from build123d import *

# Parameters (mm, degrees)
SALIENTE_EXTRUIR1_DEPTH = 50
CROQUIS3_R              = 1.75
CORTAR_EXTRUIR1_DEPTH   = 50
CORTAR_EXTRUIR2_DEPTH   = 50
CROQUIS5_W              = 13.75
CROQUIS5_H              = 15.668518787
SALIENTE_EXTRUIR2_DEPTH = 5
CROQUIS6_R              = 3.25
CORTAR_EXTRUIR3_DEPTH   = 51


with BuildPart() as part:
    # Croquis1 → Saliente-Extruir1 (new body)
    with BuildSketch(Plane.XY):
        Polygon((-11.139985082, 4.35106383), (12.860014918, 4.35106383), (8.360014918, 22.35106383), (-6.639985082, 22.35106383), align=None)
        Polygon((-6.068188312, 13.064935956), (-2.604086697, 7.064935956), (4.324116534, 7.064935956), (7.788218149, 13.064935956), (4.324116534, 19.064935956), (-2.604086697, 19.064935956), align=None, mode=Mode.SUBTRACT)
    extrude(amount=SALIENTE_EXTRUIR1_DEPTH)

    # Croquis3 → Cortar-Extruir1 (cut)
    with BuildSketch(Plane.XZ.offset(-4.35106383)):
        with Locations((-8.139985082, 3.5)):
            Circle(CROQUIS3_R)
        with Locations((9.860014918, 46.5)):
            Circle(CROQUIS3_R)
    extrude(amount=-CORTAR_EXTRUIR1_DEPTH, mode=Mode.SUBTRACT)

    # Croquis4 → Cortar-Extruir2 (cut)
    with BuildSketch(Plane(origin=(0, 7.35106383, 0), x_dir=(-1, 0, 0), z_dir=(0, -1, 0))):
        with BuildLine():
            Line((-18.110014918, -43.75), (-9.860014918, -43.75))
            ThreePointArc((-9.860014918, -43.75), (-7.91547127, -44.555456352), (-7.110014918, -46.5))
            Line((-7.110014918, -46.5), (-7.110014918, -54.75))
            Line((-7.110014918, -54.75), (-18.110014918, -54.75))
            Line((-18.110014918, -54.75), (-18.110014918, -43.75))
        make_face()
        with BuildLine():
            Line((16.389985082, -6.25), (8.139985082, -6.25))
            ThreePointArc((8.139985082, -6.25), (6.195441433, -5.444543648), (5.389985082, -3.5))
            Line((5.389985082, -3.5), (5.389985082, 4.75))
            Line((5.389985082, 4.75), (16.389985082, 4.75))
            Line((16.389985082, 4.75), (16.389985082, -6.25))
        make_face()
    extrude(amount=-CORTAR_EXTRUIR2_DEPTH, mode=Mode.SUBTRACT)

    # Croquis5 → Saliente-Extruir2 (add)
    with BuildSketch(Plane.XY.offset(50)):
        with Locations((0.235014918, 14.516804437)):
            Rectangle(CROQUIS5_W, CROQUIS5_H)
    extrude(amount=-SALIENTE_EXTRUIR2_DEPTH)

    # Croquis6 → Cortar-Extruir3 (cut, through all)
    with BuildSketch(Plane(origin=(0, 0, 0), x_dir=(-1, 0, 0), z_dir=(0, 0, -1))):
        with Locations((-0.860014918, 12.564935956)):
            Circle(CROQUIS6_R)
    extrude(amount=-CORTAR_EXTRUIR3_DEPTH, mode=Mode.SUBTRACT)


solid = part.part
Design review of the part built by this model. Coordinates are the model's own, in mm. A direction names the side the tool comes from. Coordinates: 2 decimals unless noted, no trailing zeros. Loops run counter-clockwise (first coordinate to the right, second up) from the corner with the lowest first, then second, coordinate; pieces in that order, holes last. Notation, with made-up numbers: (82, 64) -> (118, 64) arc R30 cw to (118, 101) -> close; hole circle Ø4 at (-9.5, 89). An arc over 180 degrees is marked (long way). Use a Markdown table: item, result. Add a question column.
Item 1: Wall thickness on L1, parallel to Y at x = -2.5, z = 34; L2, parallel to Z at x = -3, y = 12.75; L3, parallel to Z at x = -8.75, y = 12.5: over which ranges is each line inside the solid? List them lowest first. Write a range as from..to.
Item 2: We need section A-A, the plane z = 30.5. Write out the cut boundary in (x, y).
Item 3: We need section B-B, the plane y = 11.25. Write out the cut boundary in (x, z).
Item 4: We need section D-D, the plane y = 8.5. Write out the cut boundary in (x, z).
Item 5: Machinability: for faces 1 (the flat face through (9, 7.351, 48.2)), 2 (the flat face through (1, 22.351, 25)), 3 (the flat face through (6.03, 10.02, 22.92)), 4 (the flat face through (-5.39, 10, 2)), which of the approach directions +Z, -Z, +X, -X, +Y, -Y give a long, thin tool a straight path to every point of the face, cutting with its end or side? Answer none if there is none.
Item 6: The part is to be moulded in two halves that separate along X. For faces 5 (the flat face through (-9, 10, 6.25)), 6 (the flat face through (-4.36, 10.11, 22.18)), 7 (the cylindrical face through (7.94, 14.75, 44.53)), say which applies: +X half, -X half, draft (parallel to the pull), parting line (faces both ways), or undercut.
Item 7: Clearance check with flat-ended pins moving along their axes: P1, Ø4, axis at y = 15, z = 46.5, coming from the +X side; P2, Ø1, axis at y = 20, z = 22, coming from the -X side; P3, Ø0.7, axis at x = 11.5, y = 11.5, coming from the +Z side; P4, Ø7.5, axis at x = 0.86, y = 12.56, coming from the -Z side. State where each tip first meets the part, or that it passes through.
Item 8: We need section C-C, the plane x = 1.5. Write out the cut boundary in (y, z).
Numbers:
| question | item | result |
|---|---|---|
| 1 | L1 | y = 4.35..7.06, 19.06..22.35 |
| 1 | L2 | z = 45..50 |
| 1 | L3 | z = 6.25..50 |
| 2 | outline | (-11.14, 4.35) -> (12.86, 4.35) -> (8.36, 22.35) -> (-6.64, 22.35) -> close; hole (-6.07, 13.06) -> (-2.6, 7.06) -> (4.32, 7.06) -> (7.79, 13.06) -> (4.32, 19.06) -> (-2.6, 19.06) -> close |
| 3 | outline | (-9.42, 6.25) -> (-8.14, 6.25) arc R2.75 cw to (-5.39, 3.5) -> (-5.39, 0) -> (-5.02, 0) -> (-5.02, 45) -> (-2.11, 45) -> (-2.11, 50) -> (-9.42, 50) -> close; (3.83, 45) -> (6.74, 45) -> (6.74, 0) -> (11.14, 0) -> (11.14, 43.75) -> (9.86, 43.75) arc R2.75 cw to (7.11, 46.5) -> (7.11, 50) -> (3.83, 50) -> close |
| 4 | outline | (-10.1, 6.25) -> (-8.14, 6.25) arc R2.75 cw to (-5.39, 3.5) -> (-5.39, 0) -> (-3.43, 0) -> (-3.43, 45) -> (5.15, 45) -> (5.15, 0) -> (11.82, 0) -> (11.82, 43.75) -> (9.86, 43.75) arc R2.75 cw to (7.11, 46.5) -> (7.11, 50) -> (-10.1, 50) -> close |
| 5 | face 1 | +Z, +X, +Y |
| 5 | face 2 | +Z, -Z, +X, -X, +Y |
| 5 | face 3 | -Z |
| 5 | face 4 | -Z, -X, +Y |
| 6 | face 5 | draft |
| 6 | face 6 | undercut |
| 6 | face 7 | +X half |
| 7 | P1 | stops at x = 7.97 |
| 7 | P2 | stops at x = -7.35 |
| 7 | P3 | passes through |
| 7 | P4 | stops at z = 45 |
| 8 | outline | (4.35, 0) -> (7.06, 0) -> (7.06, 45) -> (9.38, 45) -> (9.38, 50) -> (4.35, 50) -> close; (15.75, 45) -> (19.06, 45) -> (19.06, 0) -> (22.35, 0) -> (22.35, 50) -> (15.75, 50) -> close |
